Autodesk Inventor part; units mm, degrees
ref_plane "YZ Plane" through (0, 0, 0) normal (1, 0, 0) x (0, 1, 0)
ref_plane "XZ Plane" through (0, 0, 0) normal (0, 1, 0) x (-1, 0, 0)
ref_plane "XY Plane" through (0, 0, 0) normal (0, 0, 1) x (1, 0, 0)
sketch "Szkic1" plane through (0, 0, 0) normal (1, 0, 0) x (0, 1, 0)
  line L0 (0, 0) -> (0, -2.3094)
  line L1 (0, -2.3094) -> (23, -15.5885)
  line L2 (24.75, -14.2894) -> (0, 0)
  line L3 (23, -15.5885) -> (24.75, -15.5885)
  line L4 (24.75, -15.5885) -> (24.75, -14.2894)
  dimension "d0" = 60
  dimension "d1" = 2
  dimension "d2" = 1.75
  dimension "d3" = 23
extrude "Wyciągnięcie proste1" add sketch "Szkic1" along normal blind 98
sketch "Szkic2" plane through (98, 24.75, -15.5885) normal (0, 0, -1) x (-1, 0, 0)
  line L0 (98, -24.75) -> (0, -24.75) construction
  line L1 (12.5, -24.75) -> (36.5, -24.75)
  line L2 (36.5, -24.75) -> (36.5, -12.75)
  line L3 (36.5, -12.75) -> (12.5, -12.75)
  line L4 (12.5, -12.75) -> (12.5, -24.75)
  line L5 (49, -24.75) -> (49, 0) construction
  line L6 (98, 0) -> (0, 0) construction
  line L7 (85.5, -24.75) -> (61.5, -24.75)
  line L8 (61.5, -24.75) -> (61.5, -12.75)
  line L9 (61.5, -12.75) -> (85.5, -12.75)
  line L10 (85.5, -12.75) -> (85.5, -24.75)
  line L11 (0, -24.75) -> (0, -1.75) construction
  dimension "d6" = 12
  dimension "d7" = 24
  dimension "d8" = 12.5
extrude "Wyciągnięcie proste2" cut sketch "Szkic2" against normal through all
sketch "Szkic3" plane through (0, 24.75, -14.2894) normal (0, 0.5, 0.8660254) x (1, 0, 0)
  line L0 (0, -28.5788) -> (12.5, -28.5788) construction
  line L1 (2.4, -28.5788) -> (2.4, -14.6241) construction
  line L2 (0, 0) -> (0, -28.5788) construction
  line L3 (0, -27.4241) -> (12.5, -27.4241) construction
  line L4 (36.5, -28.5788) -> (61.5, -28.5788) construction
  line L5 (49, -28.5788) -> (49, 0.6495) construction
  line L6 (0, 0.6495) -> (98, 0.6495) construction
  point P0 (2.4, -21.1241)
  point P1 (95.6, -14.6241)
  point P2 (95.6, -21.1241)
  dimension "d11" = 2.4
  dimension "d12" = 6.3
  dimension "d13" = 12.8
hole "Otwór1" at (2.4, 12.0851, -6.9774) at (2.4, 6.456, -3.7274) at (95.6, 12.0851, -6.9774) at (95.6, 6.456, -3.7274) direction (0, -0.5, -0.8660254) diameter 3.2 depth 5 tip angle 118 countersink diameter 6.3 countersink angle 84.225
properties part number "Przod" material "Aluminium 6061"
Could you check a few things on this model? Use its own coordinates, in mm. A direction names the side the tool comes from. Round coordinates to 2 decimals unless told otherwise and drop trailing zeros. Write each loop counter-clockwise with the first axis right and the second up, starting at its lowest first coordinate (ties: lowest second). Pieces come first, ordered by that corner, then holes. Notation, with made-up numbers: M -5,21.5 L 16,21.5 A25 ccw 16,47.5 Z; hole C -25.75,-13 d8. An arc over 180 degrees is marked long. Write each question's results on one line, items separated by ' | '. Start each with the question number.
1. I need wall thicknesses on L1, parallel to Z at x = 11, y = 2.25; L2, parallel to Z at x = 36, y = 17; L3, parallel to Y at x = 47.5, z = -12. Which ranges of each line are inside material? Lowest first, please. Write a range as from..to.
2. Imagine slicing it at C-C on x = 79.5. List the corners of the cut face in (y, z) for me.
3. Thinking about a two-plate mould opening in X: for faces 1 (the face through (6, 0, -1)), 2 (the face through (93.78, 11.73, -8.41)), 3 (the face through (0, 12.3, -8.3)), 4 (the face through (3.55, 6.74, -5.74)), which applies, +X half, -X half, draft (parallel to the pull), parting line (faces both ways), or undercut?
4. I'm going to push flat-ended pins straight in: pin 1 Ø2 at (x, z) = (30, -9) entering from +Y; pin 2 Ø2.5 at (x, z) = (77, -7.5) entering from -Y; pin 3 Ø1.5 at (x, z) = (75.5, -8) entering from +Y. Where does each tip first touch, or does it pass through?
5. Imagine slicing it at A-A on x = 45. List the corners of the cut face in (y, z) for me, and give its area (3 significant figures).
6. Imagine slicing it at B-B on z = -11.75. List the corners of the cut face in (x, y) for me.
7. Imagine slicing it at D-D on y = 19.75. List the corners of the cut face in (x, z) for me.
8. On a 3-axis mill with a long thin cutter (end or side, diameter ignored), from which of +Z, -Z, +X, -X, +Y, -Y can I reach the whole of each face in a straight line? I mean faces 5 (the face through (73, 12, -8)), 6 (the face through (48.314, 15.298, -8.832)). Say none if no direction works.
Result sheet:
1) L1: z = -3.61..-1.3 | L2: z = -12.12..-9.81 | L3: y = 16.78..20.78
2) outline: M 12,-9.24 L 23,-15.59 L 24.75,-15.59 L 24.75,-14.29 L 12,-6.93 Z
3) face 1: draft | face 2: undercut | face 3: -X half | face 4: undercut
4) pin 1: stops at y = 17.32 | pin 2: stops at y = 12 | pin 3: stops at y = 15.16
5) outline: M 0,-2.31 L 23,-15.59 L 24.75,-15.59 L 24.75,-14.29 L 0,0 Z | area: 56.3 mm^2
6) outline: M 0,16.35 L 98,16.35 L 98,20.35 L 0,20.35 Z
7) outline: M 0,-13.71 L 98,-13.71 L 98,-11.4 L 0,-11.4 Z
8) face 5: +Z, -Z, -Y | face 6: +Z, +X, -X, +Y
